Design review of the part built by this model. Coordinates are the model's own, in mm. Face numbers are marked on the shaded views. A direction names the side the tool comes from. Coordinates: 2 decimals unless noted, no trailing zeros. Loops run counter-clockwise (first coordinate to the right, second up) from the corner with the lowest first, then second, coordinate; pieces in that order, holes last. Notation, with made-up numbers: M 79,65.25 L 99,65.25 A24 ccw 99,100.25 Z; hole C 23,-4.75 d3. An arc over 180 degrees is marked long. One line per item, written item: value.
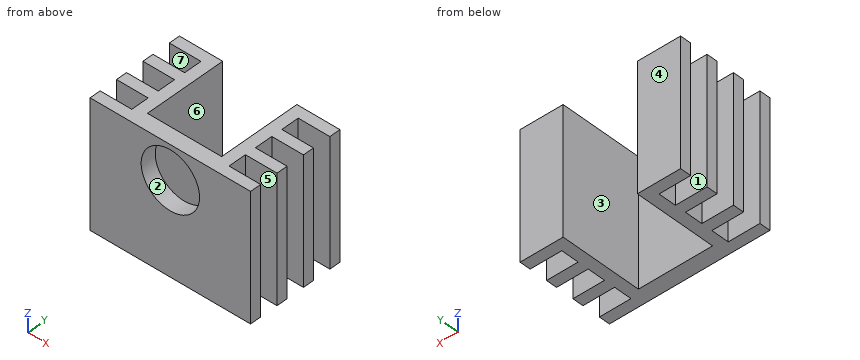
```python
from build123d import *

# Parameters (mm, degrees)
SKETCH1_W           = 33
SKETCH1_H           = 26
SKETCH1_R           = 6
BOSS_EXTRUDE1_DEPTH = 20
SKETCH2_W           = 6.5
SKETCH2_H           = 3.666666667
SKETCH2_H_2         = 3.666666666
SKETCH2_W_2         = 15.25
SKETCH2_H_3         = 16.85
CUT_EXTRUDE1_DEPTH  = 26


with BuildPart() as part:
    # Sketch1 → Boss-Extrude1 (new body)
    with BuildSketch(Plane(origin=(0, 0, 0), x_dir=(1, 0, 0), z_dir=(0, 1, 0))):
        with Locations((16.5, 13)):
            Rectangle(SKETCH1_W, SKETCH1_H)
        with Locations((16.5, 7)):
            Circle(SKETCH1_R, mode=Mode.SUBTRACT)
    extrude(amount=BOSS_EXTRUDE1_DEPTH)

    # Sketch2 → Cut-Extrude1 (cut)
    with BuildSketch(Plane.XY):
        with Locations((3.25, 4.083333334)):
            Rectangle(SKETCH2_W, SKETCH2_H)
        with Locations((3.25, 10)):
            Rectangle(SKETCH2_W, SKETCH2_H_2)
        with Locations((3.25, 15.916666666)):
            Rectangle(SKETCH2_W, SKETCH2_H)
        with Locations((29.75, 15.916666666)):
            Rectangle(SKETCH2_W, SKETCH2_H)
        with Locations((29.75, 10)):
            Rectangle(SKETCH2_W, SKETCH2_H_2)
        with Locations((29.75, 4.083333334)):
            Rectangle(SKETCH2_W, SKETCH2_H)
        with Locations((16.525, 11.575)):
            Rectangle(SKETCH2_W_2, SKETCH2_H_3)
    extrude(amount=-CUT_EXTRUDE1_DEPTH, mode=Mode.SUBTRACT)


solid = part.part
```
(1) Mouldability with a two-part tool opening along X and no side actions: class the marked faces 1, 2 and 3 as released by +X, released by -X, zero draft, split by the parting line, or undercut.
Reply:
face 1: zero draft
face 2: undercut
face 3: undercut
(2) We need section B-B on x = 31. State the section outline as (y, z) points.
Reply:
outline: M 0,-26 L 2.25,-26 L 2.25,0 L 0,0 Z; M 5.92,-26 L 8.17,-26 L 8.17,0 L 5.92,0 Z; M 11.83,-26 L 14.08,-26 L 14.08,0 L 11.83,0 Z; M 17.75,-26 L 20,-26 L 20,0 L 17.75,0 Z
(3) We need section C-C on x = 16.5. State the section outline as (y, z) points, then the cut area to 3 significant figures.
Reply:
outline: M 0,-26 L 3.15,-26 L 3.15,-13 L 0,-13 Z; M 0,-1 L 3.15,-1 L 3.15,0 L 0,0 Z
area: 44.1 mm2
(4) Tool access review of the marked faces 4, 5, 6 and 7: name each direction out of +Z, -Z, +X, -X, +Y, -Y from which nothing blocks a thin tool from reaching the whole face with its end or side.
Reply:
face 4: +Z, -Z, +X, -X, +Y
face 5: +Z, -Z, +X
face 6: +Z, -Z, +Y
face 7: +Z, -Z, -X
(5) We need section A-A on y = 4. State the section outline as (x, z) points.
Reply:
outline: M 6.5,-26 L 8.9,-26 L 8.9,0 L 6.5,0 Z; M 24.15,-26 L 26.5,-26 L 26.5,0 L 24.15,0 Z
(6) To check wall thickness, follow line 1 along Y through (x, z) = (4, -20.5); line 2 along X through (y, z) = (0.7, -7); line 3 along X through (y, z) = (8, -2.75). State the ranges of each line that lie inside material, in increasing order. Write a range as [from, to].
Reply:
line 1: y = [0, 2.25], [5.92, 8.17], [11.83, 14.08], [17.75, 20]
line 2: x = [0, 10.5], [22.5, 33]
line 3: x = [0, 8.9], [24.15, 33]
(7) Insertion check: pin 1 (8.5 mm diameter, centred on y = 7.5, z = -17, fed in from -X); pin 2 (1.1 mm diameter, centred on y = 11, z = -13.5, fed in from -X); pin 3 (4.5 mm diameter, centred on x = 13, z = -15, fed in from +Y). Each pin has a flat end and moves straight along its axis. Give the tip position at first contact, or say it passes through.
Reply:
pin 1: stops at x = 0
pin 2: stops at x = 6.5
pin 3: stops at y = 3.15
